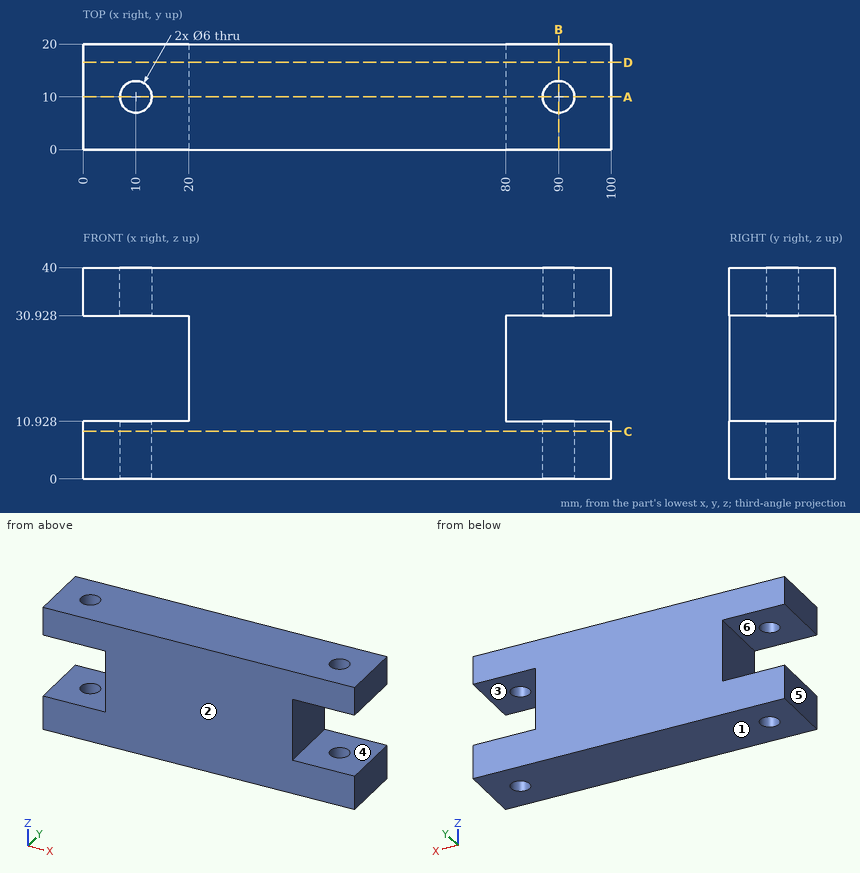
Geometry: see drawing. Coordinates: mm, zero at the bounding-box minimum. A direction names the side the tool comes from. Give positions to 0.01 mm unless a question says otherwise; leave off trailing zeros. Order: outer loops, then holes, each group sorted by start corner. A loop starts at its lowest first (then second) coordinate and runs counter-clockwise, first axis right, second up. Notation, with made-up numbers: M 4.25,66 L 55.25,66 A18 ccw 55.25,86 Z; hole C -39,87 d7. An arc over 180 degrees is marked long. Answer as a JSON object with one key per item and string values.
1. First-contact query: P1, Ø6, axis at y = 6, z = 22.5, coming from the +X side; P2, Ø4, axis at y = 16, z = 13.5, coming from the -X side. Flat tips, straight axial feed; report the tip coordinate or a pass-through.
Result sheet:
{"P1": "x = 80", "P2": "x = 20"}
2. Cut plane B-B, the plane x = 90. Output: boundary loops of the cut face in (y, z), and give its area (3 significant figures).
Result sheet:
{"outline": "M 0,0 L 7,0 L 7,10.93 L 0,10.93 Z; M 0,30.93 L 7,30.93 L 7,40 L 0,40 Z; M 13,0 L 20,0 L 20,10.93 L 13,10.93 Z; M 13,30.93 L 20,30.93 L 20,40 L 13,40 Z", "area": "280 mm²"}
3. Reachability of the marked faces 4, 5 and 6 from +Z, -Z, +X, -X, +Y, -Y: full face, straight path, thin tool, end or side. Return the list, or none.
Result sheet:
{"face 4": "+X, +Y, -Y", "face 5": "+Z, -Z, -X, +Y, -Y", "face 6": "-X, +Y, -Y"}
4. Cut plane C-C, the plane z = 9. Output: boundary loops of the cut face in (x, y), and give its area (3 significant figures).
Result sheet:
{"outline": "M 0,0 L 100,0 L 100,20 L 0,20 Z; hole C 10,10 d6; hole C 90,10 d6", "area": "1,940 mm²"}
5. Pull-direction query (Z, two-part tool) for the marked faces 1, 2 and 3; classes: +Z half, -Z half, draft (parallel to the pull), parting line (faces both ways), or undercut.
Result sheet:
{"face 1": "-Z half", "face 2": "draft", "face 3": "undercut"}
6. Cut plane D-D, the plane y = 16.5. Output: boundary loops of the cut face in (x, z).
Result sheet:
{"outline": "M 0,0 L 100,0 L 100,10.93 L 80,10.93 L 80,30.93 L 100,30.93 L 100,40 L 0,40 L 0,30.93 L 20,30.93 L 20,10.93 L 0,10.93 Z"}
7. Cut plane A-A, the plane y = 10. Output: boundary loops of the cut face in (x, z), and give its area (3 significant figures).
Result sheet:
{"outline": "M 0,0 L 7,0 L 7,10.93 L 0,10.93 Z; M 0,30.93 L 7,30.93 L 7,40 L 0,40 Z; M 13,0 L 87,0 L 87,10.93 L 80,10.93 L 80,30.93 L 87,30.93 L 87,40 L 13,40 L 13,30.93 L 20,30.93 L 20,10.93 L 13,10.93 Z; M 93,0 L 100,0 L 100,10.93 L 93,10.93 Z; M 93,30.93 L 100,30.93 L 100,40 L 93,40 Z", "area": "2,960 mm²"}
8. Ray query, line 1 (Z direction, x = 18.5, y = 14.25); line 2 (X direction, y = 7.5, z = 38.5) (1 decimal); line 3 (Y direction, x = 90, z = 7). Return the intervals inside material, ascending. Write a range as [from, to].
Result sheet:
{"line 1": "[0, 10.93], [30.93, 40]", "line 2": "[0, 8.3], [11.7, 88.3], [91.7, 100]", "line 3": "[0, 7], [13, 20]"}
